```python
from build123d import *

# Parameters (mm, degrees)
CROQUIS1_R                     = 21.825
SALIENTE_EXTRUIR1_DEPTH        = 4.5
CROQUIS2_R                     = 2.75
SALIENTE_EXTRUIR2_DEPTH        = 12
TALADRO_DE_MARGEN_PARA_M121_D  = 13.5
SALIENTE_EXTRUIR3_DEPTH        = 12
CROQUIS8_R                     = 1.7
CORTAR_EXTRUIR1_DEPTH          = 16.5
MATRIZC1_COUNT                 = 3
TALADRO_DE_MARGEN_PARA_M2_51_D = 2.9
SALIENTE_EXTRUIR5_DEPTH        = 4.5
MATRIZC2_COUNT                 = 3
CROQUIS12_R                    = 2.875
CORTAR_EXTRUIR2_DEPTH          = 2.2
CROQUIS13_R                    = 3.1
CORTAR_EXTRUIR3_DEPTH          = 2
CROQUIS14_R                    = 3.1
CORTAR_EXTRUIR4_DEPTH          = 3.5


with BuildPart() as part:
    # Croquis1 → Saliente-Extruir1 (new body)
    with BuildSketch(Plane(origin=(0, 0, 0), x_dir=(1, 0, 0), z_dir=(0, 1, 0))):
        Circle(CROQUIS1_R)
    extrude(amount=SALIENTE_EXTRUIR1_DEPTH)

    # Croquis2 → Saliente-Extruir2 (add)
    with BuildSketch(Plane(origin=(0, 4.5, 0), x_dir=(1, 0, 0), z_dir=(0, 1, 0))):
        with Locations((0, 15)):
            Circle(CROQUIS2_R)
        with Locations((12.990381057, -7.5)):
            Circle(CROQUIS2_R)
        with Locations((-12.990381057, -7.5)):
            Circle(CROQUIS2_R)
    extrude(amount=SALIENTE_EXTRUIR2_DEPTH)

    # Taladro de margen para M121 (through all)
    with Locations(Plane(origin=(0, 4.5, 0), x_dir=(1, 0, 0), z_dir=(0, 1, 0))):
        with Locations((0, 0)):
            Hole(TALADRO_DE_MARGEN_PARA_M121_D / 2)

    # Croquis5 → Saliente-Extruir3 (add)
    with BuildSketch(Plane(origin=(0, 4.5, 0), x_dir=(1, 0, 0), z_dir=(0, 1, 0))):
        with BuildLine():
            ThreePointArc((-7.642674188, 4.4125), (-11.035446071, 10.994501306), (-11.800237164, 18.359875487))
            ThreePointArc((-11.800237164, 18.359875487), (-18.901004438, 10.9125), (-21.800237164, 1.039367411))
            ThreePointArc((-21.800237164, 1.039367411), (-15.039240468, 4.059725986), (-7.642674188, 4.4125))
        make_face()
    saliente_extruir3 = extrude(amount=SALIENTE_EXTRUIR3_DEPTH)

    # Croquis8 → Cortar-Extruir1 (cut)
    with BuildSketch(Plane(origin=(0, 16.5, 0), x_dir=(1, 0, 0), z_dir=(0, 1, 0))):
        with Locations((-14.722431864, 8.5)):
            Circle(CROQUIS8_R)
    cortar_extruir1 = extrude(amount=-CORTAR_EXTRUIR1_DEPTH, mode=Mode.SUBTRACT)

    # MatrizC1: Saliente-Extruir3, Cortar-Extruir1 ×3 about axis
    matrizc1_axis = Axis((0, 0, 0), (0, 1, 0))
    for i in range(1, MATRIZC1_COUNT):
        add(saliente_extruir3.rotate(matrizc1_axis, i * 360 / MATRIZC1_COUNT))
        add(cortar_extruir1.rotate(matrizc1_axis, i * 360 / MATRIZC1_COUNT), mode=Mode.SUBTRACT)

    # Taladro de margen para M2.51 (through all)
    with Locations(Plane(origin=(0, 16.5, 0), x_dir=(1, 0, 0), z_dir=(0, 1, 0))):
        with Locations((12.990381057, -7.5), (-12.990381057, -7.5), (0, 15)):
            Hole(TALADRO_DE_MARGEN_PARA_M2_51_D / 2)

    # Croquis11 → Saliente-Extruir5 (add)
    with BuildSketch(Plane.XZ):
        with BuildLine():
            ThreePointArc((-10, 19.399242898), (-18.901004438, 10.9125), (-21.800237164, -1.039367411))
            ThreePointArc((-21.800237164, -1.039367411), (-23.615858472, 13.634622246), (-10, 19.399242898))
        make_face()
    saliente_extruir5 = extrude(amount=-SALIENTE_EXTRUIR5_DEPTH)

    # MatrizC2: Saliente-Extruir5 ×3 about axis
    matrizc2_axis = Axis((0, 0, 0), (0, 1, 0))
    for i in range(1, MATRIZC2_COUNT):
        add(saliente_extruir5.rotate(matrizc2_axis, i * 360 / MATRIZC2_COUNT))

    # Croquis12 → Cortar-Extruir2 (cut)
    with BuildSketch(Plane.XZ):
        with Locations((-12.990381057, 7.5)):
            Circle(CROQUIS12_R)
        with Locations((12.990381057, 7.5)):
            Circle(CROQUIS12_R)
        with Locations((0, -15)):
            Circle(CROQUIS12_R)
    extrude(amount=-CORTAR_EXTRUIR2_DEPTH, mode=Mode.SUBTRACT)

    # Croquis13 → Cortar-Extruir3 (cut)
    with BuildSketch(Plane(origin=(0, 16.5, 0), x_dir=(1, 0, 0), z_dir=(0, 1, 0))):
        with Locations((0, -17)):
            Circle(CROQUIS13_R)
        with Locations((-14.722431864, 8.5)):
            Circle(CROQUIS13_R)
        with Locations((14.722431864, 8.5)):
            Circle(CROQUIS13_R)
    extrude(amount=-CORTAR_EXTRUIR3_DEPTH, mode=Mode.SUBTRACT)

    # Croquis14 → Cortar-Extruir4 (cut)
    with BuildSketch(Plane.XZ):
        with Locations((-14.722431864, -8.5)):
            Circle(CROQUIS14_R)
    extrude(amount=-CORTAR_EXTRUIR4_DEPTH, mode=Mode.SUBTRACT)


solid = part.part
```
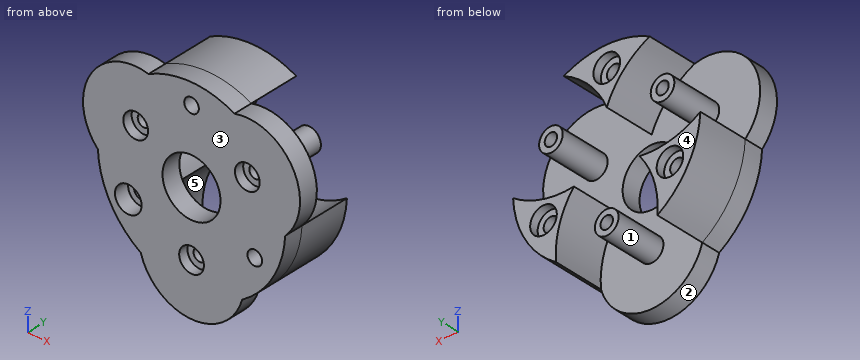
Read the model definition and answer for the solid it produces. Units are mm, in the model's axes. Face numbers are marked on the shaded views. A direction names the side the tool comes from. Round coordinates to 2 decimals unless told otherwise and drop trailing zeros. Write each loop counter-clockwise with the first axis right and the second up, starting at its lowest first coordinate (ties: lowest second). Pieces come first, ordered by that corner, then holes. Notation, with made-up numbers: (-33, 84) - (-22, 84) arc R35 cw to (-22, 118) - close; hole circle Ø7 at (68.5, 51). An arc over 180 degrees is marked (long way). Use CSV: the item, a comma, the result in double quotes.
Q1. Find section D-D, the plane x = 19. Write down the section's boundary in (y, z).
Values:
outline,"(0, -10.74) - (16.5, -10.74) - (16.5, -2.66) - (4.5, -2.66) - (4.5, 18.2) - (0, 18.2) - close"
Q2. Find section C-C, the plane z = 17. Write down the section's boundary in (x, y), then the cut area to 3 significant figures.
Values:
outline,"(-20.75, 0) - (-1.7, 0) - (-1.7, 14.5) - (-3.1, 14.5) - (-3.1, 16.5) - (-6.13, 16.5) - (-6.13, 4.5) - (-20.75, 4.5) - close; (1.7, 0) - (20.75, 0) - (20.75, 4.5) - (6.13, 4.5) - (6.13, 16.5) - (3.1, 16.5) - (3.1, 14.5) - (1.7, 14.5) - close"
area,"272 mm²"
Q3. Find section A-A, the plane y = 7.25. Count the separate pieces of the cut face and the enclosed holes in it, then the cut area to 3 significant figures.
Values:
separate pieces,"6"
enclosed holes,"6"
area,"359 mm²"
Q4. Find section B-B, the plane z = 7.5. Write down the section's boundary in (x, y), then the cut area to 3 significant figures.
Values:
outline,"(-25.26, 0) - (-15.87, 0) - (-15.87, 2.2) - (-14.44, 2.2) - (-14.44, 16.5) - (-15.74, 16.5) - (-15.74, 4.5) - (-25.26, 4.5) - close; (-11.54, 2.2) - (-10.12, 2.2) - (-10.12, 0) - (10.12, 0) - (10.12, 2.2) - (11.54, 2.2) - (11.54, 16.5) - (10.24, 16.5) - (10.24, 4.5) - (-10.24, 4.5) - (-10.24, 16.5) - (-11.54, 16.5) - close; (14.44, 2.2) - (15.87, 2.2) - (15.87, 0) - (25.26, 0) - (25.26, 4.5) - (15.74, 4.5) - (15.74, 16.5) - (14.44, 16.5) - close"
area,"251 mm²"
Q5. Straight lines are drawn through the part: line 1 along X through (y, z) = (6.75, 7.5); line 2 along X through (y, z) = (6, -15); line 3 along Y through (x, z) = (-11, 11.5). For each, find the intervals that lie inside material, in ascending order.
Values:
line 1,"x = -15.74 to -14.44, -11.54 to -10.24, 10.24 to 11.54, 14.44 to 15.74"
line 2,"x = -15.85 to -11.8, -2.75 to -1.45, 1.45 to 2.75, 11.8 to 15.85"
line 3,"y = 0 to 4.5"
Q6. A tool of negligible diameter and unlimited length cuts with its end or side. For the marked faces 4 and 5, from which of +Z, -Z, +X, -X, +Y, -Y can it reach the whole face along a straight path? Write none if from no direction.
Values:
face 4,"+Z, -Z, +X, -X, +Y"
face 5,"+Y"
Q7. Each of these flat-tipped pins is pushed along its axis until it touches: pin 1 Ø3 at (x, z) = (0.5, 17.5) entering from +Y; pin 2 Ø5 at (x, z) = (-14.72, -8.5) entering from -Y; pin 3 Ø5 at (y, z) = (6.5, 16) entering from +X. Where does it stop, or does it pass through?
Values:
pin 1,"stops at y = 14.5"
pin 2,"stops at y = 3.5"
pin 3,"stops at x = 23.07"
Q8. Determine the mould class of the marked faces 1, 2 and 3 for opening direction X: +X half, -X half, draft (parallel to the pull), parting line (faces both ways), or undercut.
Values:
face 1,"undercut"
face 2,"parting line"
face 3,"draft"
